Can you work these out from the model? Positions are in its coordinate system, mm. Face numbers are marked on the shaded views. A direction names the side the tool comes from. Coordinates: 2 decimals unless noted, no trailing zeros. Order: outer loops, then holes, each group sorted by start corner. A loop starts at its lowest first (then second) coordinate and runs counter-clockwise, first axis right, second up. Notation, with made-up numbers: M -37,-3.5 L 17,-3.5 A33 cw 17,34.5 Z; hole C -10,-18.5 d11. An arc over 180 degrees is marked long. Answer as CSV lines item,"result". Start each with the question number.
1. If we section it at A-A (x = 0): List the corners of the cut face in (y, z) for me.
2. If we section it at C-C (y = -4.75): List the corners of the cut face in (x, z) for me.
3. If we mould it in two halves opening along Y, with no side actions, what happens to the marked faces 1, 2, 3 and 4? For each: released by +Y, released by -Y, zero draft, split by the parting line, or undercut.
4. If we section it at D-D (x = -1.75): List the corners of the cut face in (y, z) for me, plus the area to 3 significant figures.
5. Will these pins go through, and if not, where does the flat tip stop? pin 1 (2 mm diameter, centred on y = -4.5, z = 2.5, fed in from -X); pin 2 (1.5 mm diameter, centred on y = 0.5, z = 4.5, fed in from +X); pin 3 (3 mm diameter, centred on x = -1.5, z = 2, fed in from -Y).
6. On a 3-axis mill with a long thin cutter (end or side, diameter ignored), from which of +Z, -Z, +X, -X, +Y, -Y can I reach the whole of each face in a straight line? I mean the marked faces 5 and 6. Say none if no direction works.
7. I need wall thicknesses on line 1 along Y through (x, z) = (0, -0.4); line 2 along X through (y, z) = (0, -0.55); line 3 along Z through (x, y) = (-6.5, -0.5). Which ranges of each line are inside material? Lowest first, please. Write a range as from..to.
8. If we section it at B-B (z = 3.5): List the corners of the cut face in (x, y) for me.
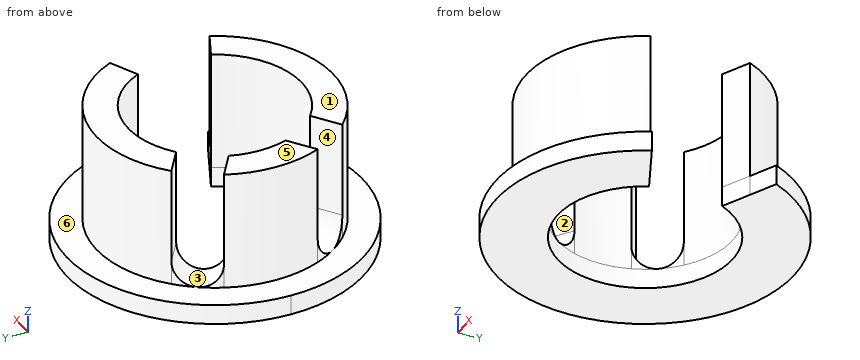
```python
from build123d import *

# Parameters (mm, degrees)
BOSS_EXTRUDE1_DEPTH = 6
BOSS_EXTRUDE2_START = 1
BOSS_EXTRUDE2_DEPTH = 1
CUT_EXTRUDE1_START  = -6
CUT_EXTRUDE1_DEPTH  = 6
FILLET1_R           = 1.2


with BuildPart() as part:
    # Sketch1 → Boss-Extrude1 (new body)
    with BuildSketch(Plane.XY):
        with BuildLine():
            Line((3.987754263, 1.859520352), (5.437846722, 2.53570957))
            ThreePointArc((5.437846722, 2.53570957), (-6, 0), (5.437846722, -2.53570957))
            Line((5.437846722, -2.53570957), (3.987754263, -1.859520352))
            ThreePointArc((3.987754263, -1.859520352), (-4.4, 0), (3.987754263, 1.859520352))
        make_face()
    extrude(amount=BOSS_EXTRUDE1_DEPTH)

    # Sketch2 → Boss-Extrude2 (add)
    with BuildSketch(Plane(origin=(0, 0, 0), x_dir=(-1, 0, 0), z_dir=(0, 0, -1)).offset(BOSS_EXTRUDE2_START)):
        with BuildLine():
            Line((-3.987754263, -1.859520352), (-5.437846722, -2.53570957))
            ThreePointArc((-5.437846722, -2.53570957), (6, 0), (-5.437846722, 2.53570957))
            Line((-5.437846722, 2.53570957), (-3.987754263, 1.859520352))
            ThreePointArc((-3.987754263, 1.859520352), (4.4, 0), (-3.987754263, -1.859520352))
        make_face()
        with BuildLine():
            Line((-6.797308403, 3.169636963), (-5.437846722, 2.53570957))
            ThreePointArc((-5.437846722, 2.53570957), (6, 0), (-5.437846722, -2.53570957))
            Line((-5.437846722, -2.53570957), (-6.797308403, -3.169636963))
            ThreePointArc((-6.797308403, -3.169636963), (1.623297105, -7.322220053), (7.5, 0))
            ThreePointArc((7.5, 0), (1.623297105, 7.322220053), (-6.797308403, 3.169636963))
        make_face()
    extrude(amount=-BOSS_EXTRUDE2_DEPTH)

    # Sketch3 → Cut-Extrude1 (cut)
    with BuildSketch(Plane.XY.offset(6).offset(CUT_EXTRUDE1_START)):
        with BuildLine():
            ThreePointArc((-5.503902596, -2.388944581), (-4.914912266, -3.441458618), (-4.127319149, -4.354909487))
            Line((-4.127319149, -4.354909487), (-2.779344429, -3.411047427))
            ThreePointArc((-2.779344429, -3.411047427), (-3.604268995, -2.52373632), (-4.155927876, -1.44508252))
            Line((-4.155927876, -1.44508252), (-5.503902596, -2.388944581))
        make_face()
        with BuildLine():
            ThreePointArc((-5.376200178, 5.229385398), (-6.143640332, 4.301823273), (-6.752783625, 3.263420492))
            Line((-6.752783625, 3.263420492), (-5.503902596, 2.388944581))
            ThreePointArc((-5.503902596, 2.388944581), (-4.914912266, 3.441458618), (-4.127319149, 4.354909487))
            Line((-4.127319149, 4.354909487), (-5.376200178, 5.229385398))
        make_face()
        with BuildLine():
            ThreePointArc((-4.127319149, 4.354909487), (-4.914912266, 3.441458618), (-5.503902596, 2.388944581))
            Line((-5.503902596, 2.388944581), (-4.155927876, 1.44508252))
            ThreePointArc((-4.155927876, 1.44508252), (-3.604268995, 2.52373632), (-2.779344429, 3.411047427))
            Line((-2.779344429, 3.411047427), (-4.127319149, 4.354909487))
        make_face()
        with BuildLine():
            ThreePointArc((-6.752783625, -3.263420492), (-6.143640332, -4.301823273), (-5.376200178, -5.229385398))
            Line((-5.376200178, -5.229385398), (-4.127319149, -4.354909487))
            ThreePointArc((-4.127319149, -4.354909487), (-4.914912266, -3.441458618), (-5.503902596, -2.388944581))
            Line((-5.503902596, -2.388944581), (-6.752783625, -3.263420492))
        make_face()
    extrude(amount=CUT_EXTRUDE1_DEPTH, mode=Mode.SUBTRACT)

    # Fillet1
    # the kernel refuses this fillet: 1.2 mm, written as the material it adds along each edge
    with BuildSketch(Plane(origin=(-6.584775282, -6.075638796, 0), x_dir=(-0.5735764363510464, 0.8191520442889915, 0), z_dir=(0.8191520442889916, 0.5735764363510465, 0))) as fillet1_piece_1_section:
        with BuildLine():
            CenterArc((FILLET1_R, FILLET1_R), FILLET1_R, 180, 90)
            Line((0, FILLET1_R), (0, 0))
            Line((0, 0), (FILLET1_R, 0))
        make_face()
    fillet1_piece_1 = extrude(amount=7.645573285, mode=Mode.PRIVATE)
    fillet1_piece_1 = fillet1_piece_1 - Plane(origin=(0, 0, 0.272987172), x_dir=(0.9063077870366507, 0.4226182617406977, 0), z_dir=(0, 0, -1)) * Cylinder(4.4, 21, mode=Mode.PRIVATE)
    fillet1_piece_1 = fillet1_piece_1 & Plane(origin=(0, 0, 0.272987172), x_dir=(0.9063077870366507, 0.4226182617406977, 0), z_dir=(0, 0, -1)) * Cylinder(6, 21, mode=Mode.PRIVATE)
    add(fillet1_piece_1)
    with BuildSketch(Plane(origin=(-1.698471743, 0.275646789, 0), x_dir=(0.5735764363510474, -0.8191520442889908, 0), z_dir=(-0.819152044288991, -0.5735764363510474, 0))) as fillet1_piece_2_section:
        with BuildLine():
            CenterArc((FILLET1_R, FILLET1_R), FILLET1_R, 180, 90)
            Line((0, FILLET1_R), (0, 0))
            Line((0, 0), (FILLET1_R, 0))
        make_face()
    fillet1_piece_2 = extrude(amount=7.645573285, mode=Mode.PRIVATE)
    fillet1_piece_2 = fillet1_piece_2 - Plane(origin=(0, 0, 0.272986937), x_dir=(0.9063077870366507, 0.4226182617406977, 0), z_dir=(0, 0, -1)) * Cylinder(4.4, 21, mode=Mode.PRIVATE)
    fillet1_piece_2 = fillet1_piece_2 & Plane(origin=(0, 0, 0.272986937), x_dir=(0.9063077870366507, 0.4226182617406977, 0), z_dir=(0, 0, -1)) * Cylinder(6, 21, mode=Mode.PRIVATE)
    add(fillet1_piece_2)
    with BuildSketch(Plane(origin=(-0.321888296, 1.690318118, 0), x_dir=(0, 0, 1), z_dir=(-0.8191520442889906, 0.5735764363510478, 0))) as fillet1_piece_3_section:
        with BuildLine():
            CenterArc((FILLET1_R, -FILLET1_R), FILLET1_R, 90, 90)
            Line((0, -FILLET1_R), (0, 0))
            Line((0, 0), (FILLET1_R, 0))
        make_face()
    fillet1_piece_3 = extrude(amount=7.645573285, mode=Mode.PRIVATE)
    fillet1_piece_3 = fillet1_piece_3 - Plane(origin=(0, 0, 0.272987798), x_dir=(0.9063077870366507, -0.4226182617406978, 0), z_dir=(0, 0, -1)) * Cylinder(4.4, 21, mode=Mode.PRIVATE)
    fillet1_piece_3 = fillet1_piece_3 & Plane(origin=(0, 0, 0.272987798), x_dir=(0.9063077870366507, 0.4226182617406977, 0), z_dir=(0, 0, -1)) * Cylinder(6, 21, mode=Mode.PRIVATE)
    add(fillet1_piece_3)
    with BuildSketch(Plane(origin=(-1.698471743, -0.275646789, 0), x_dir=(0.5735764363510463, 0.8191520442889917, 0), z_dir=(-0.8191520442889917, 0.5735764363510463, 0))) as fillet1_piece_4_section:
        with BuildLine():
            CenterArc((FILLET1_R, -FILLET1_R), FILLET1_R, 90, 90)
            Line((0, -FILLET1_R), (0, 0))
            Line((0, 0), (FILLET1_R, 0))
        make_face()
    fillet1_piece_4 = extrude(amount=7.645573285, mode=Mode.PRIVATE)
    fillet1_piece_4 = fillet1_piece_4 - Plane(origin=(0, 0, 0.27298714), x_dir=(0.9063077870366507, 0.4226182617406977, 0), z_dir=(0, 0, -1)) * Cylinder(4.4, 21, mode=Mode.PRIVATE)
    fillet1_piece_4 = fillet1_piece_4 & Plane(origin=(0, 0, 0.27298714), x_dir=(0.9063077870366507, 0.4226182617406977, 0), z_dir=(0, 0, -1)) * Cylinder(6, 21, mode=Mode.PRIVATE)
    add(fillet1_piece_4)


solid = part.part
```
Solved:
1,outline,"M -7.5,-1 L -4.4,-1 L -4.4,6 L -6,6 L -6,0 L -7.5,0 Z; M 4.4,-1 L 7.5,-1 L 7.5,0 L 6,0 L 6,6 L 4.4,6 Z"
2,outline,"M -5.8,-1 L 5.8,-1 L 5.8,0 L 3.67,0 L 3.67,6 L -3.67,6 L -3.67,0 L -5.8,0 Z"
3,face 1,"zero draft"
3,face 2,"released by -Y"
3,face 3,"undercut"
3,face 4,"undercut"
4,outline,"M -7.29,-1 L -4.04,-1 L -4.04,6 L -5.74,6 L -5.74,0 L -7.29,0 Z; M 4.04,-1 L 7.29,-1 L 7.29,0 L 5.74,0 L 5.74,6 L 4.04,6 Z"
4,area,"26.9 mm²"
5,pin 1,"x = -4.13"
5,pin 2,"x = -4.22"
5,pin 3,"y = -6"
6,face 5,"+Z, +X, -X, +Y, -Y"
6,face 6,"+Z"
7,line 1,"-7.5..-4.4, 4.4..7.5"
7,line 2,"-7.5..-4.4"
7,line 3,"-1..0"
8,outline,"M -5.5,-2.39 L -4.16,-1.45 A4.4 cw -4.16,1.45 L -5.5,2.39 A6 ccw Z; M -4.13,-4.35 A6 ccw 5.44,-2.54 L 3.99,-1.86 A4.4 cw -2.78,-3.41 Z; M -4.13,4.35 L -2.78,3.41 A4.4 cw 3.99,1.86 L 5.44,2.54 A6 ccw Z"
